Source: CAD feature listing. Evaluate the final solid. Frame: model axes, mm. A direction names the side the tool comes from. Give positions to 0.01 mm unless a question says otherwise; leave off trailing zeros. Order: outer loops, then holes, each group sorted by start corner. A loop starts at its lowest first (then second) coordinate and runs counter-clockwise, first axis right, second up. Notation, with made-up numbers: M -22.75,-23 L 18.25,-23 A22 ccw 18.25,5 Z; hole C 43,49 d2. An arc over 180 degrees is marked long. Answer as a JSON object with one key per item and string values. Group by question number.
1. Section query D-D (x = 12.5). Output: boundary loops of the cut face in (y, z) (3 decimals).
2. Pin query (flat end, axial travel): P1, Ø10, axis at x = -3, z = 57, coming from the +Y side; P2, Ø1.5, axis at x = -4, z = 50, coming from the +Y side; P3, Ø2, axis at x = 2, z = 59.5, coming from the +Y side; P4, Ø4.5, axis at x = 7, y = -8.1, coming from the +Z side. Return the tip coordinate at first contact, or that it passes through.
3. Section query C-C (z = 30.5). Output: boundary loops of the cut face in (x, y) (3 decimals).
4. Section query A-A (x = 0). Output: boundary loops of the cut face in (y, z) (3 decimals), plus the area to 3 significant figures.
5. Pull-direction query (X, two-part tool) for faces 6 (the flat face through (0.21, -1.427, 3.076)), 7 (the flat face through (8.388, -5.651, 54.028)); classes: +X half, -X half, draft (parallel to the pull), parting line (faces both ways), or undercut.
6. Material intervals for L1, parallel to Z at x = -8.5, y = -4.6; L2, parallel to Z at x = -2, y = -4.6; L3, parallel to X at y = -8.1, z = 58.85, sorted ascending. Write a range as [from, to].
7. Set-up query: faces 1 (the flat face through (-13.028, 4.606, 47.86)), 2 (the flat face through (-8.3, -9.5, 55.6)), 3 (the cylindrical face through (-0.1, -7.5, 57.5)), 4 (the cylindrical face through (-6.95, -9.85, 58.64)), 5 (the flat face through (0, -0.35, 0)). Return all of +Z, -Z, +X, -X, +Y, -Y with unobstructed straight access to the full face (end or side cutting, diameter ignored); none if empty.
8. Section query B-B (y = -8.1). Count the separate pieces of the cut face and the enclosed holes in it, plus the area to 3 significant figures.
from build123d import *
from build123d.topology import SkipClean

# Parameters (mm, degrees)
SCHIZZO7_W                    = 30
SCHIZZO7_H                    = 24.2
ESTRUSIONE_ESTRUSIONE3_DEPTH  = 7.5
TAGLIO_ESTRUSIONE1_REACH      = 35.206
SCHIZZO12_W                   = 30
SCHIZZO12_H                   = 9
ESTRUSIONE_ESTRUSIONE5_DEPTH  = 54.1
TAGLIO_ESTRUSIONE3_REACH      = 67.197
SCHIZZO15_W                   = 22
SCHIZZO15_H                   = 18
TAGLIO_ESTRUSIONE4_DEPTH      = 8.3
TAGLIO_ESTRUSIONE5_REACH      = 73.737
TAGLIO_ESTRUSIONE6_DEPTH      = 3.1
SCHIZZO20_W                   = 30
SCHIZZO20_H                   = 15.2
ESTRUSIONE_ESTRUSIONE6_DEPTH  = 27
ESTRUSIONE_ESTRUSIONE7_DEPTH  = 4
ESTRUSIONE_ESTRUSIONE8_DEPTH  = 4
ESTRUSIONE_ESTRUSIONE9_DEPTH  = 1
ESTRUSIONE_ESTRUSIONE10_START = -13.1
ESTRUSIONE_ESTRUSIONE10_DEPTH = 1


# Read off the part's stored shape, not the designer's step: Estrusione-Estrusione10
with BuildPart() as part:
    # Schizzo7 → Estrusione-Estrusione3 (new, symmetric)
    with BuildSketch(Plane.XY):
        Rectangle(SCHIZZO7_W, SCHIZZO7_H)
        with BuildLine():
            Line((2.453738644, 8.85), (-2.453738644, 8.85))
            Line((-2.453738644, 8.85), (-3.680607966, 6.725))
            ThreePointArc((-3.680607966, 6.725), (0, 0.35), (3.680607966, 6.725))
            Line((3.680607966, 6.725), (2.453738644, 8.85))
        make_face(mode=Mode.SUBTRACT)
    extrude(amount=ESTRUSIONE_ESTRUSIONE3_DEPTH, both=True)

    # Schizzo8 → Taglio-Estrusione1 (cut, up to next)
    with BuildSketch(Plane(origin=(15, 0, 0), x_dir=(0, 0, -1), z_dir=(1, 0, 0)), mode=Mode.PRIVATE) as taglio_estrusione1_sk1:
        with BuildLine():
            Line((-2.453738644, -0.35), (2.453738644, -0.35))
            Line((2.453738644, -0.35), (3.680607966, -2.475))
            ThreePointArc((3.680607966, -2.475), (0, -8.85), (-3.680607966, -2.475))
            Line((-3.680607966, -2.475), (-2.453738644, -0.35))
        make_face()
    taglio_estrusione1_tool1 = extrude(taglio_estrusione1_sk1.sketch, amount=-TAGLIO_ESTRUSIONE1_REACH, mode=Mode.PRIVATE) & part.part
    add(taglio_estrusione1_tool1.solids().sort_by_distance((15, -4.474132, 0))[0], mode=Mode.SUBTRACT)

    # Schizzo12 → Estrusione-Estrusione5 (add)
    with BuildSketch(Plane.XY.offset(7.5)):
        with Locations((0, -7.6)):
            Rectangle(SCHIZZO12_W, SCHIZZO12_H)
    extrude(amount=ESTRUSIONE_ESTRUSIONE5_DEPTH)

    # Schizzo14 → Taglio-Estrusione3 (cut, up to next)
    with BuildSketch(Plane(origin=(0, -3.1, 0), x_dir=(1, 0, 0), z_dir=(0, 1, 0)), mode=Mode.PRIVATE) as taglio_estrusione3_sk1:
        with BuildLine():
            Line((4.1, -61.6), (-4.1, -61.6))
            ThreePointArc((-4.1, -61.6), (0, -57.5), (4.1, -61.6))
        make_face()
    taglio_estrusione3_tool1 = extrude(taglio_estrusione3_sk1.sketch, amount=-TAGLIO_ESTRUSIONE3_REACH, mode=Mode.PRIVATE) & part.part
    add(taglio_estrusione3_tool1.solids().sort_by_distance((0, -3.1, 59.859906))[0], mode=Mode.SUBTRACT)

    # Schizzo15 → Taglio-Estrusione4 (cut)
    with BuildSketch(Plane(origin=(0, -3.1, 0), x_dir=(1, 0, 0), z_dir=(0, 1, 0))):
        with Locations((0, -43.5)):
            Rectangle(SCHIZZO15_W, SCHIZZO15_H)
    extrude(amount=-TAGLIO_ESTRUSIONE4_DEPTH, mode=Mode.SUBTRACT)

    # Schizzo16 → Taglio-Estrusione5 (cut, up to next)
    with BuildSketch(Plane.XY.offset(61.6), mode=Mode.PRIVATE) as taglio_estrusione5_sk1:
        with BuildLine():
            Line((-8.010362971, -6.35), (-5.989637029, -6.35))
            Line((-5.989637029, -6.35), (-5.484455543, -7.225))
            ThreePointArc((-5.484455543, -7.225), (-7, -9.85), (-8.515544457, -7.225))
            Line((-8.515544457, -7.225), (-8.010362971, -6.35))
        make_face()
    taglio_estrusione5_tool1 = extrude(taglio_estrusione5_sk1.sketch, amount=-TAGLIO_ESTRUSIONE5_REACH, mode=Mode.PRIVATE) & part.part
    # Schizzo16 → Taglio-Estrusione5 (cut, up to next)
    with BuildSketch(Plane.XY.offset(61.6), mode=Mode.PRIVATE) as taglio_estrusione5_sk2:
        with BuildLine():
            Line((5.989637029, -6.35), (8.010362971, -6.35))
            Line((8.010362971, -6.35), (8.515544457, -7.225))
            ThreePointArc((8.515544457, -7.225), (7, -9.85), (5.484455543, -7.225))
            Line((5.484455543, -7.225), (5.989637029, -6.35))
        make_face()
    taglio_estrusione5_tool2 = extrude(taglio_estrusione5_sk2.sketch, amount=-TAGLIO_ESTRUSIONE5_REACH, mode=Mode.PRIVATE) & part.part
    add(taglio_estrusione5_tool1.solids().sort_by_distance((-7, -8.048172, 61.6))[0], mode=Mode.SUBTRACT)
    add(taglio_estrusione5_tool2.solids().sort_by_distance((7, -8.048172, 61.6))[0], mode=Mode.SUBTRACT)

    # Schizzo17 → Taglio-Estrusione6 (cut)
    with BuildSketch(Plane(origin=(0, 0, 52.5), x_dir=(-1, 0, 0), z_dir=(0, 0, -1))):
        Polygon((-7, -11.35), (-4.185417438, -9.725), (-4.185417438, -6.475), (-7, -4.85), (-9.814582562, -6.475), (-9.814582562, -9.725), align=None)
        Polygon((9.814582562, -9.725), (7, -11.35), (4.185417438, -9.725), (4.185417438, -6.475), (7, -4.85), (9.814582562, -6.475), align=None)
    extrude(amount=-TAGLIO_ESTRUSIONE6_DEPTH, mode=Mode.SUBTRACT)

    # Schizzo20 → Estrusione-Estrusione6 (add)
    with SkipClean():  # the faces are left unmerged after this step: merging them gives an invalid solid
        with BuildSketch(Plane.XY.offset(7.5)):
            with Locations((0, 4.5)):
                Rectangle(SCHIZZO20_W, SCHIZZO20_H)
            with BuildLine():
                Line((-2.453738644, 8.85), (2.453738644, 8.85))
                Line((2.453738644, 8.85), (3.680607966, 6.725))
                ThreePointArc((3.680607966, 6.725), (0, 0.35), (-3.680607966, 6.725))
                Line((-3.680607966, 6.725), (-2.453738644, 8.85))
            make_face(mode=Mode.SUBTRACT)
        extrude(amount=ESTRUSIONE_ESTRUSIONE6_DEPTH)

    # Schizzo21 → Estrusione-Estrusione7 (add)
    with SkipClean():  # the faces are left unmerged after this step: merging them gives an invalid solid
        with BuildSketch(Plane.ZY.offset(15)):
            Polygon((34.5, 12.1), (61.6, -3.1), (34.5, -3.1), align=None)
        extrude(amount=-ESTRUSIONE_ESTRUSIONE7_DEPTH)

    # Schizzo22 → Estrusione-Estrusione8 (add)
    with SkipClean():  # the faces are left unmerged after this step: merging them gives an invalid solid
        with BuildSketch(Plane(origin=(15, 0, 0), x_dir=(0, 0, -1), z_dir=(1, 0, 0))):
            Polygon((-34.5, 12.1), (-61.6, -3.1), (-34.5, -3.1), align=None)
        extrude(amount=-ESTRUSIONE_ESTRUSIONE8_DEPTH)

    # Schizzo24 → Estrusione-Estrusione9 (add)
    with SkipClean():  # the faces are left unmerged after this step: merging them gives an invalid solid
        with BuildSketch(Plane.XZ.offset(12.1)):
            with BuildLine():
                Line((15, 61.6), (4.1, 61.6))
                ThreePointArc((4.1, 61.6), (0, 57.5), (-4.1, 61.6))
                Line((-4.1, 61.6), (-15, 61.6))
                Line((-15, 61.6), (-15, -7.5))
                Line((-15, -7.5), (15, -7.5))
                Line((15, -7.5), (15, 61.6))
            make_face()
        extrude(amount=ESTRUSIONE_ESTRUSIONE9_DEPTH)

    # Estrusione-Estrusione10 outline → Estrusione-Estrusione10 (add)
    with SkipClean():  # the faces are left unmerged after this step: merging them gives an invalid solid
        with BuildSketch(Plane(origin=(0, 0, 0), x_dir=(1, 0, 0), z_dir=(0, 1, 0)).offset(ESTRUSIONE_ESTRUSIONE10_START)):
            with BuildLine():
                Line((-4.1, -61.6), (4.1, -61.6))
                ThreePointArc((4.1, -61.6), (0, -57.5), (-4.1, -61.6))
            make_face()
        extrude(amount=ESTRUSIONE_ESTRUSIONE10_DEPTH)


solid = part.part
Answer sheet:
{
 "1": {"outline": "M -13.1,-7.5 L 12.1,-7.5 L 12.1,34.5 L -3.1,61.6 L -13.1,61.6 Z; hole M -2.475,-3.681 L -0.35,-2.454 L -0.35,2.454 L -2.475,3.681 A4.25 ccw long Z"},
 "2": {"P1": "y = -3.1", "P2": "y = -11.4", "P3": "y = -12.1", "P4": "z = 61.6"},
 "3": {"outline": "M -15,-13.1 L 15,-13.1 L 15,12.1 L -15,12.1 Z; hole M -3.681,6.725 A4.25 ccw long 3.681,6.725 L 2.454,8.85 L -2.454,8.85 Z"},
 "4": {"outline": "M -13.1,-7.5 L 0.35,-7.5 L 0.35,34.5 L -11.4,34.5 L -11.4,52.5 L -3.1,52.5 L -3.1,57.5 L -12.1,57.5 L -12.1,61.6 L -13.1,61.6 Z; M 8.85,-7.5 L 12.1,-7.5 L 12.1,34.5 L 8.85,34.5 Z; hole M -2.475,-3.681 L -0.35,-2.454 L -0.35,2.454 L -2.475,3.681 A4.25 ccw long Z", "area": "727 mm^2"},
 "5": {"face 6": "draft", "face 7": "undercut"},
 "6": {"L1": "[-7.5, -4.25], [4.25, 34.5], [52.5, 61.6]", "L2": "[-7.5, -4.25], [4.25, 34.5], [52.5, 58.02]", "L3": "[-15, -8.75], [-5.25, -3.04], [3.04, 5.25], [8.75, 15]"},
 "7": {"face 1": "+Z, +X, -X, +Y", "face 2": "none", "face 3": "+Z, +Y", "face 4": "+Z", "face 5": "+X, -X"},
 "8": {"separate pieces": "3", "enclosed holes": "0", "area": "1,430 mm^2"}
}
